Source: CAD feature listing. Evaluate the final solid. Frame: model axes, mm. Face numbers are marked on the shaded views. A direction names the side the tool comes from. Round coordinates to 2 decimals unless told otherwise and drop trailing zeros.
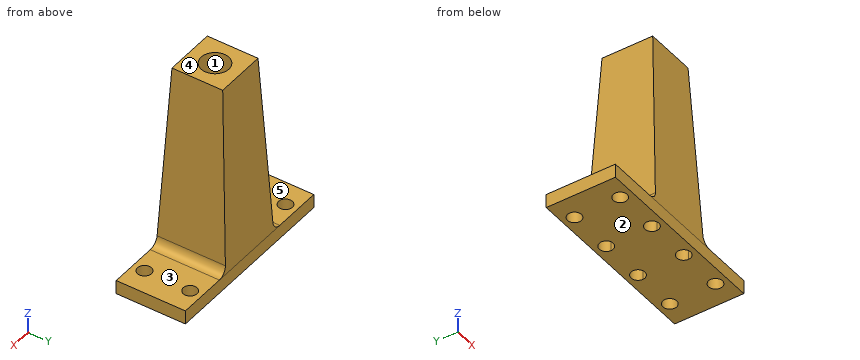
from build123d import *

# Parameters (mm, degrees)
SKETCH_1_W          = 40
SKETCH_1_H          = 15
SKETCH_1_R          = 1.5
EXTRUDE_1_DEPTH     = 3
SKETCH_5_R          = 1.5
CUT_EXTRUDE_3_DEPTH = 8
SKETCH_8_R          = 2.999642866
CUT_EXTRUDE_4_DEPTH = 15
SKETCH_9_R          = 1.5
CUT_EXTRUDE_5_DEPTH = 15
FILLET_1_R          = 2


with BuildPart() as part:
    # 草图1 → 凸台-拉伸1 (new body)
    with BuildSketch(Plane.XY):
        Rectangle(SKETCH_1_W, SKETCH_1_H)
        with Locations((4.95, 4.95)):
            Circle(SKETCH_1_R, mode=Mode.SUBTRACT)
        with Locations((4.95, -4.95)):
            Circle(SKETCH_1_R, mode=Mode.SUBTRACT)
        with Locations((-4.95, -4.95)):
            Circle(SKETCH_1_R, mode=Mode.SUBTRACT)
        with Locations((-4.95, 4.95)):
            Circle(SKETCH_1_R, mode=Mode.SUBTRACT)
    extrude(amount=EXTRUDE_1_DEPTH)

    # 草图3 → 放样1 section 0
    with BuildSketch(Plane.XY.offset(43)):
        with BuildLine():
            Line((-5.5, -5.5), (5.5, -5.5))
            Line((5.5, -5.5), (5.5, 5.5))
            Line((5.5, 5.5), (-5.5, 5.5))
            Line((-5.5, 5.5), (-5.5, -5.5))
        make_face()
    # 草图2 → 放样1 section 1
    with BuildSketch(Plane.XY.offset(3)):
        with BuildLine():
            Line((-7.5, -7.5), (7.5, -7.5))
            Line((7.5, -7.5), (7.5, 7.5))
            Line((7.5, 7.5), (-7.5, 7.5))
            Line((-7.5, 7.5), (-7.5, -7.5))
        make_face()
    loft()

    # 草图5 → 切除-拉伸3 (cut)
    with BuildSketch(Plane(origin=(0, 0, 0), x_dir=(-1, 0, 0), z_dir=(0, 0, -1))):
        with Locations((4.95, -4.95)):
            Circle(SKETCH_5_R)
        with Locations((4.95, 4.95)):
            Circle(SKETCH_5_R)
        with Locations((-4.95, 4.95)):
            Circle(SKETCH_5_R)
        with Locations((-4.95, -4.95)):
            Circle(SKETCH_5_R)
    extrude(amount=-CUT_EXTRUDE_3_DEPTH, mode=Mode.SUBTRACT)

    # 草图8 → 切除-拉伸4 (cut)
    with BuildSketch(Plane.XY.offset(43)):
        Circle(SKETCH_8_R)
    extrude(amount=-CUT_EXTRUDE_4_DEPTH, mode=Mode.SUBTRACT)

    # 草图9 → 切除-拉伸5 (cut)
    with BuildSketch(Plane(origin=(0, 0, 0), x_dir=(-1, 0, 0), z_dir=(0, 0, -1))):
        with Locations((-14.848989873, -4.95)):
            Circle(SKETCH_9_R)
        with Locations((-14.848989873, 4.949494936)):
            Circle(SKETCH_9_R)
        with Locations((14.849494937, 4.949494936)):
            Circle(SKETCH_9_R)
        with Locations((14.849494937, -4.95)):
            Circle(SKETCH_9_R)
    extrude(amount=-CUT_EXTRUDE_5_DEPTH, mode=Mode.SUBTRACT)

    # 圆角1
    fillet_1_edges = [part.edges().sort_by_distance(p)[0] for p in [
        (7.5, 0, 3),
        (-7.5, 0, 3),
    ]]
    fillet(fillet_1_edges, radius=FILLET_1_R)


solid = part.part
1) Reachability of the marked faces 3, 4 and 5 from +Z, -Z, +X, -X, +Y, -Y: full face, straight path, thin tool, end or side. Return the list, or none.
Taken from the geometry:
face 3: +Z, +X, +Y, -Y
face 4: +Z, +X, -X, +Y, -Y
face 5: +Z, -X, +Y, -Y
2) Material intervals for line 1 (Y direction, x = -4, z = 4); line 2 (X direction, y = 4.95, z = 5.6); line 3 (X direction, y = 4, z = 7), sorted ascending.
Taken from the geometry:
line 1: y = -7.45 to -6.11, -3.79 to 3.79, 6.11 to 7.45
line 2: x = -7.37 to -6.45, -3.45 to 3.45, 6.45 to 7.37
line 3: x = -7.3 to -6.11, -3.79 to 3.79, 6.11 to 7.3
3) Contact query for flat-ended pins moving along their axis: P1, Ø0.9, axis at x = 4.5, y = 5.5, coming from the -Z side; P2, Ø5, axis at y = -2.5, z = 9, coming from the -X side (3 decimals); P3, Ø8.5, axis at x = -16, y = -1.5, coming from the +Z side; P4, Ø2.5, axis at x = 14.85, y = 4.95, coming from the +Z side. Output: stop coordinate, or through.
Taken from the geometry:
P1: stops at z = 8
P2: stops at x = -7.325
P3: stops at z = 3
P4: passes through
4) Pull-direction query (X, two-part tool) for the marked faces 1 and 2; classes: released by +X, released by -X, zero draft, split by the parting line, or undercut.
Taken from the geometry:
face 1: undercut
face 2: zero draft
